from build123d import *

# Parameters (mm, degrees)
F0_W     = 50
F0_H     = 70
F1_DEPTH = 15
F2_T     = 1.2
F3_W     = 52.4
F3_H     = 72.4
F3_W_2   = 50.8
F3_H_2   = 70.8
F4_DEPTH = 5
F5_R     = 1
F6_W     = 10
F6_H     = 10
F7_DEPTH = 25


with BuildPart() as f1:
    # F0 (on Top) → F1 (new body)
    with BuildSketch(Plane.XY):
        with Locations((25, 35)):
            Rectangle(F0_W, F0_H)
    extrude(amount=F1_DEPTH)

    # F2
    f2_openings = [f1.faces().sort_by_distance(p)[0] for p in [
        (25, 35, 15),
    ]]
    offset(amount=F2_T, openings=f2_openings, kind=Kind.INTERSECTION)

    # F3 (on face) → F4 (cut)
    with BuildSketch(Plane.XY.offset(15)):
        with Locations((25, 35)):
            Rectangle(F3_W, F3_H)
        with Locations((25, 35)):
            Rectangle(F3_W_2, F3_H_2, mode=Mode.SUBTRACT)
    extrude(amount=-F4_DEPTH, mode=Mode.SUBTRACT)

    # F5
    f5_edges = [f1.edges().sort_by_distance(p)[0] for p in [
        (-1.2, 71.2, 4.4),
        (-1.2, -1.2, 4.4),
        (51.2, -1.2, 4.4),
        (51.2, 71.2, 4.4),
    ]]
    fillet(f5_edges, radius=F5_R)

    # F6 (on face) → F7 (cut)
    with BuildSketch(Plane.XZ.offset(1.2)):
        with Locations((25, 15)):
            Rectangle(F6_W, F6_H)
    extrude(amount=-F7_DEPTH, mode=Mode.SUBTRACT)


solid = f1.part
Here's how the part is built. I have some questions about the finished solid (model axes, mm). A direction names the side the tool comes from. Coordinates: 2 decimals unless noted, no trailing zeros. Order: outer loops, then holes, each group sorted by start corner. A loop starts at its lowest first (then second) coordinate and runs counter-clockwise, first axis right, second up. Notation, with made-up numbers: (47.25, -18) -> (60.25, -18) arc R20 cw to (60.25, 10) -> close; hole circle Ø5 at (-33.5, -26). An arc over 180 degrees is marked (long way). Answer in a Markdown table with one row per item.
(1) I want a section at C-C on z = 8.25. List the corners of the cut face in (x, y) for me.
Answer key:
| item | result |
|---|---|
| outline | (-1.2, -0.2) arc R1 ccw to (-0.2, -1.2) -> (50.2, -1.2) arc R1 ccw to (51.2, -0.2) -> (51.2, 70.2) arc R1 ccw to (50.2, 71.2) -> (-0.2, 71.2) arc R1 ccw to (-1.2, 70.2) -> close; hole (0, 0) -> (50, 0) -> (50, 70) -> (0, 70) -> close |
(2) I want a section at A-A on z = 12.75. List the corners of the cut face in (x, y) for me.
Answer key:
| item | result |
|---|---|
| outline | (-0.4, -0.4) -> (20, -0.4) -> (20, 0) -> (0, 0) -> (0, 70) -> (50, 70) -> (50, 0) -> (30, 0) -> (30, -0.4) -> (50.4, -0.4) -> (50.4, 70.4) -> (-0.4, 70.4) -> close |
(3) Please list where these lines run through material, in increasing order: probe 1 along Y at (x, z) = (17.5, 10.5); probe 2 along Y at (x, z) = (33.5, 3); probe 3 along X at (y, z) = (40, 8.25).
Answer key:
| item | result |
|---|---|
| probe 1 | -0.4 to 0, 70 to 70.4 |
| probe 2 | -1.2 to 0, 70 to 71.2 |
| probe 3 | -1.2 to 0, 50 to 51.2 |
(4) Will these pins go through, and if not, where does the flat tip stop? pin 1 Ø5.5 at (x, z) = (34, 13.5) entering from +Y; pin 2 Ø12 at (x, y) = (41, 40.5) entering from +Z; pin 3 Ø2.5 at (y, z) = (45, 12) entering from +X.
Answer key:
| item | result |
|---|---|
| pin 1 | y = 70.4 |
| pin 2 | z = 0 |
| pin 3 | x = 50.4 |
(5) I want a section at B-B on y = 23. List the corners of the cut face in (x, z) for me, then the cut area to 3 significant figures.
Answer key:
| item | result |
|---|---|
| outline | (-1.2, -1.2) -> (51.2, -1.2) -> (51.2, 10) -> (50.4, 10) -> (50.4, 15) -> (50, 15) -> (50, 0) -> (0, 0) -> (0, 15) -> (-0.4, 15) -> (-0.4, 10) -> (-1.2, 10) -> close |
| area | 90.9 mm^2 |
(6) I want a section at D-D on x = 22.5. List the corners of the cut face in (y, z) for me, then the cut area to 3 significant figures.
Answer key:
| item | result |
|---|---|
| outline | (-1.2, -1.2) -> (71.2, -1.2) -> (71.2, 10) -> (70.4, 10) -> (70.4, 15) -> (70, 15) -> (70, 0) -> (0, 0) -> (0, 10) -> (-1.2, 10) -> close |
| area | 113 mm^2 |
(7) Thinking about a two-plate mould opening in Y: for faces 5 (the face through (25, 70, 7)), 6 (the face through (10, -0.4, 13)), 7 (the face through (25, 70.4, 13)), which applies, +Y half, -Y half, draft (parallel to the pull), parting line (faces both ways), or undercut?
Answer key:
| item | result |
|---|---|
| face 5 | undercut |
| face 6 | -Y half |
| face 7 | +Y half |
(8) On a 3-axis mill with a long thin cutter (end or side, diameter ignored), from which of +Z, -Z, +X, -X, +Y, -Y can I reach the whole of each face in a straight line? I mean faces 1 (the face through (50.4, 35, 13)), 2 (the face through (-0.4, 35, 13)), 3 (the face through (40, -0.4, 13)), 4 (the face through (0, 35, 7)). Say none if no direction works.
Answer key:
| item | result |
|---|---|
| face 1 | +Z, +X, +Y, -Y |
| face 2 | +Z, -X, +Y, -Y |
| face 3 | +Z, +X, -X, -Y |
| face 4 | +Z |
